```python
from build123d import *


with BuildPart() as part:
    # Esquisse1 → Révolution1 (revolve)
    with BuildSketch(Plane.XY):
        with BuildLine():
            Line((0, 0), (0, 50))
            Line((0, 50), (2, 50))
            Line((2, 50), (2, 2))
            Line((2, 2), (41.535898385, 2))
            ThreePointArc((41.535898385, 2), (46.03527618, 3.863703305), (49, 0))
            Line((49, 0), (0, 0))
        make_face()
    r_volution1 = revolve(axis=Axis((0, 0, 0), (1, 0, 0)))

    # Symétrie1: Révolution1 across plane
    add(r_volution1.mirror(Plane(origin=(0, 0, 0), x_dir=(0, 0, 1), z_dir=(1, 0, 0))))


solid = part.part
```
For this review, take the finished solid that the model builds, in its own axes (mm). Coordinates: 2 decimals unless noted, no trailing zeros. Loops run counter-clockwise (first coordinate to the right, second up) from the corner with the lowest first, then second, coordinate; pieces in that order, holes last.
1. Add section A-A, the plane y = 0. Give the boundary of the cut face in (x, z).
2. Add section D-D, the plane y = 44.5. Give the boundary of the cut face in (x, z).
3. Mouldability with a two-part tool opening along X and no side actions: class faces 1 (the cylindrical face through (22, 0, -2)), 2 (the cylindrical face through (-0.03, 47.69, 15.02)), 3 (the cylindrical face through (-22, 0, -2)) as +X half, -X half, draft (parallel to the pull), parting line (faces both ways), or undercut.
4. Add section C-C, the plane x = -22. Give the boundary of the cut face in (y, z).
5. For line 1 (X direction, y = -7.5, z = -6.5); line 2 (Z direction, x = 20.5, y = 0.5), list the stretches that pass through material, from the lowest coordinate up.
6. Insertion check: P1, Ø1.5, axis at y = 22.5, z = -28.5, coming from the +X side; P2, Ø1.5, axis at y = 32.5, z = 25.5, coming from the -X side; P3, Ø12, axis at x = 39, y = -3, coming from the +Z side. Each pin has a flat end and moves straight along its axis. Give the tip position at first contact, or say it passes through.
Result:
1. outline: (-41.54, -2) - (-2, -2) - (-2, -50) - (2, -50) - (2, -2) - (41.54, -2) arc R4 ccw (long way) to (41.54, 2) - (2, 2) - (2, 50) - (-2, 50) - (-2, 2) - (-41.54, 2) arc R4 ccw (long way) to start
2. outline: (-2, -22.8) - (2, -22.8) - (2, 22.8) - (-2, 22.8) - close
3. face 1: undercut
3. face 2: draft
3. face 3: undercut
4. outline: circle Ø4 at (0, 0)
5. line 1: x = -2 to 2
5. line 2: z = -1.94 to 1.94
6. P1: stops at x = 2
6. P2: stops at x = -2
6. P3: stops at z = 3.94
